Autodesk Inventor part; units mm, degrees
ref_plane "YZ Plane" through (0, 0, 0) normal (1, 0, 0) x (0, 1, 0)
ref_plane "XZ Plane" through (0, 0, 0) normal (0, 1, 0) x (-1, 0, 0)
ref_plane "XY Plane" through (0, 0, 0) normal (0, 0, 1) x (1, 0, 0)
ref_plane "Work Plane1" through (219.9513, -256.0439, -597.7148) normal (-0.097, -0.9551, 0.28) x (-0.203, -0.2564, -0.945)
sketch "Sketch3" plane through (219.9513, -256.0439, -597.7148) normal (-0.097, -0.9551, 0.28) x (-0.203, -0.2564, -0.945)
  line L0 (-0.0023, 59.9989) -> (-40.0023, 59.9989)
  line L1 (-0.0023, 59.9989) -> (39.9977, 59.9989) construction
  line L2 (-60.0163, -0.0152) -> (-60.0163, 39.9848)
  line L3 (-60.0163, -0.0152) -> (-20.0163, -0.0152) construction
  line L4 (-60.0163, -0.0152) -> (-0.0023, -0.0152)
  line L5 (-0.0023, -0.0152) -> (-0.0023, 59.9989)
  arc A0 (-49.9687, 64.958) -> (-40.0023, 59.9989) centre (-40.0023, 72.4933) ccw
  arc A1 (-60.0163, 39.9848) -> (-64.9755, 49.9513) centre (-72.5108, 39.9848) ccw
  arc A2 (-49.9687, 64.958) -> (-64.9755, 49.9513) centre (-58.5144, 58.4969) ccw
  line L6 (-40.0023, 59.9989) -> (-40.0023, 59.4989)
  line L7 (-60.0163, 39.9848) -> (-59.5163, 39.9848)
  arc A3 (-59.5163, 39.9848) -> (-40.0023, 59.4989) centre (-59.5163, 59.4989) ccw
  line L8 (-60.0163, -0.0152) -> (-80.0163, -0.0152)
  line L9 (-60.0163, -40.0152) -> (-59.5163, -40.0152)
  arc A4 (-64.9755, -49.9816) -> (-60.0163, -40.0152) centre (-72.5108, -40.0152) ccw
  line L10 (-60.0163, -0.0152) -> (-60.0163, -40.0152)
  arc A5 (-64.9755, -49.9816) -> (-49.9687, -64.9884) centre (-58.5144, -58.5273) ccw
  arc A6 (-40.0023, -60.0292) -> (-49.9687, -64.9884) centre (-40.0023, -72.5237) ccw
  arc A7 (-40.0023, -59.5292) -> (-59.5163, -40.0152) centre (-59.5163, -59.5292) ccw
  line L11 (-40.0023, -60.0292) -> (-40.0023, -59.5292)
  line L12 (-0.0023, -60.0292) -> (-40.0023, -60.0292)
  line L13 (-0.0023, -0.0152) -> (-0.0023, -60.0292)
  line L14 (-0.0023, 59.9989) -> (-40.0023, 59.9989) construction
  line L15 (-0.0023, 59.9989) -> (39.9977, 59.9989)
  line L16 (60.0118, -0.0152) -> (60.0118, 39.9848)
  line L17 (60.0118, 39.9848) -> (59.5118, 39.9848)
  arc A8 (64.9709, 49.9513) -> (60.0118, 39.9848) centre (72.5063, 39.9848) ccw
  line L18 (60.0118, -0.0152) -> (20.0118, -0.0152) construction
  arc A9 (64.9709, 49.9513) -> (49.9642, 64.958) centre (58.5098, 58.4969) ccw
  arc A10 (39.9977, 59.4989) -> (59.5118, 39.9848) centre (59.5118, 59.4989) ccw
  line L19 (39.9977, 59.9989) -> (39.9977, 59.4989)
  arc A11 (39.9977, 59.9989) -> (49.9642, 64.958) centre (39.9977, 72.4933) ccw
  line L20 (60.0118, -0.0152) -> (-0.0023, -0.0152)
  line L21 (60.0118, -40.0152) -> (59.5118, -40.0152)
  line L22 (60.0118, -0.0152) -> (60.0118, -40.0152)
  arc A12 (60.0118, -40.0152) -> (64.9709, -49.9816) centre (72.5063, -40.0152) ccw
  arc A13 (59.5118, -40.0152) -> (39.9977, -59.5292) centre (59.5118, -59.5292) ccw
  arc A14 (49.9642, -64.9884) -> (64.9709, -49.9816) centre (58.5098, -58.5273) ccw
  line L23 (39.9977, -60.0292) -> (39.9977, -59.5292)
  arc A15 (49.9642, -64.9884) -> (39.9977, -60.0292) centre (39.9977, -72.5237) ccw
  line L24 (-0.0023, -60.0292) -> (39.9977, -60.0292)
  line L25 (10, 10) -> (30, 10)
  line L26 (30, 10) -> (30, 40)
  line L27 (30, 40) -> (10, 40)
  line L28 (10, 40) -> (10, 10)
  line L29 (-30, -52.5) -> (-10, -52.5)
  line L30 (-10, -52.5) -> (-10, -45.5)
  line L31 (-10, -45.5) -> (-30, -45.5)
  line L32 (-30, -45.5) -> (-30, -52.5)
  ellipse E0 centre (-40.0023, 32.8682) end of major axis (-38.2648, 42.8976) minor radius 3.285
  circle A16 centre (12, 6) radius 1.5
  circle A17 centre (18, 6) radius 1.5
  circle A18 centre (24, 6) radius 1.5
  circle A19 centre (45, -22) radius 1.5
  circle A20 centre (27, -45) radius 1.5
  circle A21 centre (-25, 35) radius 1.5
  circle A22 centre (-52.5, 52.5) radius 2
  circle A23 centre (-55.5, 62.5) radius 2
  circle A24 centre (-62.5, 55.5) radius 2
  circle A25 centre (-62.5, -55.5303) radius 2
  circle A26 centre (-55.5, -62.5303) radius 2
  circle A27 centre (-52.5, -52.5303) radius 2
  circle A28 centre (52.4955, -52.5303) radius 2
  circle A29 centre (55.4955, -62.5303) radius 2
  circle A30 centre (62.4955, -55.5303) radius 2
  circle A31 centre (52.4955, 52.5) radius 2
  circle A32 centre (55.4955, 62.5) radius 2
  circle A33 centre (62.4955, 55.5) radius 2
  line L33 (52.4955, 52.5) -> (57.4955, 52.5) construction
  line L34 (48.96, 48.9645) -> (49.9642, 64.958)
  line L35 (48.96, 48.9645) -> (64.9709, 49.9513)
  line L36 (52.4955, -52.5303) -> (57.4955, -52.5303) construction
  line L37 (64.9709, -49.9816) -> (48.96, -48.9948)
  line L38 (48.96, -48.9948) -> (49.9642, -64.9884)
  line L39 (-52.5, -52.5303) -> (-47.5, -52.5303) construction
  line L40 (-49.9687, -64.9884) -> (-48.9645, -48.9948)
  line L41 (-64.9755, -49.9816) -> (-48.9645, -48.9948)
  line L42 (-52.5, 52.5) -> (-48.9645, 48.9645)
  line L43 (-52.5, 52.5) -> (-47.5, 52.5) construction
  line L44 (-48.9645, 48.9645) -> (-64.9755, 49.9513)
  line L45 (-48.9645, 48.9645) -> (-49.9687, 64.958)
  circle A34 centre (-23, -40) radius 1.5
  dimension "d14" = 40
  dimension "d15" = 180
  dimension "d16" = 40
  dimension "d17" = 90
  dimension "d18" = 12.4944
  dimension "d19" = 12.4944
  dimension "d20" = 0.5
  dimension "d21" = 0.5
  dimension "d22" = 20
  dimension "d24" = 20
  dimension "d25" = 30
  dimension "d26" = 90
  dimension "d27" = 90
  dimension "d28" = 20
  dimension "d29" = 7
  dimension "d30" = 3
  dimension "d31" = 3
  dimension "d32" = 3
  dimension "d33" = 3
  dimension "d34" = 3
  dimension "d35" = 3
  dimension "d36" = 4
  dimension "d37" = 4
  dimension "d38" = 4
  dimension "d39" = 4
  dimension "d40" = 4
  dimension "d41" = 4
  dimension "d42" = 4
  dimension "d43" = 4
  dimension "d44" = 4
  dimension "d45" = 4
  dimension "d46" = 4
  dimension "d47" = 4
  dimension "d54" = 5
  dimension "d56" = 5
  dimension "d58" = 5
  dimension "d59" = 45
  dimension "d62" = 3
extrude "Extrusion1" add sketch "Sketch3" along normal blind 4 contours L5 L4 L2 L7 A3 L6 L0 | L15 L19 A10 L17 L16 L20 L5 | L6 A3 L7 A1 L44 L45 A0 | L13 L12 L11 A7 L9 L10 L4 | L20 L22 L21 A13 L23 L24 L13 | A11 L34 L35 A8 L17 A10 L19 | L45 L44 A2 | A9 L35 L34 | L9 A7 L11 A6 L40 L41 A4 | L23 A13 L21 A12 L37 L38 A15 | L41 L40 A5 | L38 L37 A14 | A34
extrude "Extrusion3" add sketch "Sketch3" against normal blind 25 contours L45 L44 A2 | A9 L35 L34 | L41 L40 A5 | L38 L37 A14
extrude "Extrusion4" cut sketch "Sketch3" along normal blind 4 contours A34
properties part number "Ceiling" material "ABS Plastic"
The model under review builds one solid part; all positions refer to its coordinate system, in mm. A direction names the side the tool comes from. Round coordinates to 2 decimals unless told otherwise and drop trailing zeros. Loops run counter-clockwise (first coordinate to the right, second up) from the corner with the lowest first, then second, coordinate; pieces in that order, holes last. Notation, with made-up numbers: M -21.5,16 L 18.5,16 A12 ccw 18.5,21 Z; hole C 69.25,32 d10. An arc over 180 degrees is marked long. Answer as CSV lines item,"result". Start each with the question number.
Item 1: Wall thickness on line 1 (X direction, y = -257.5, z = -666); line 2 (Y direction, x = 231.5, z = -632.5); line 3 (X direction, y = -268.5, z = -614): over which ranges is each line inside the solid? List them lowest first. Write a range as [from, to].
Item 2: Mouldability with a two-part tool opening along Y and no side actions: class faces 4 (the face through (154.57, -254.19, -652.26)), 5 (the face through (155.686, -248.507, -638.288)), 6 (the face through (283.17, -240.74, -561.85)), 7 (the face through (220.69, -259.757, -595.838)) as released by +Y, released by -Y, zero draft, split by the parting line, or undercut.
Item 3: Consider section A-A (x = 210). Write out the cut boundary in (y, z).
Item 4: For faces 1 (the face through (161.334, -251.558, -646.739)), 2 (the face through (231.38, -242.45, -540.35)), 3 (the face through (286.579, -240.032, -564.035)), list the 3-axis set-ups (+Z, -Z, +X, -X, +Y, -Y) from which the entire face can be reached by the end or side of a thin tool; tool diameter is ignored.
Item 5: Insertion check: P1, Ø3, axis at x = 182, z = -611.5, coming from the -Y side; P2, Ø5, axis at x = 230.5, y = -261.5, coming from the -Z side; P3, Ø12, axis at y = -233.5, z = -545.5, coming from the -X side. Each pin has a flat end and moves straight along its axis. Give the tip position at first contact, or say it passes through.
Answer:
1,line 1,"x = [258.65, 270.14], [273.44, 277.48]"
1,line 2,"y = [-271.6, -267.41]"
1,line 3,"x = [256.28, 276.81]"
2,face 4,"undercut"
2,face 5,"released by +Y"
2,face 6,"undercut"
2,face 7,"released by -Y"
3,outline,"M -275.65,-653.76 L -271.77,-654.81 L -237.28,-537.16 L -241.16,-536.11 Z"
4,face 1,"-Z, +X"
4,face 2,"+Z, +Y"
4,face 3,"-Z"
5,P1,"stops at y = -260.88"
5,P2,"stops at z = -609.77"
5,P3,"stops at x = 166.68"
